Can you work these out from the model? Positions are in its coordinate system, mm. Face numbers are marked on the shaded views. A direction names the side the tool comes from. Give positions to 0.01 mm unless a question says otherwise; leave off trailing zeros. Loops run counter-clockwise (first coordinate to the right, second up) from the corner with the lowest first, then second, coordinate; pieces in that order, holes last.
from build123d import *

# Parameters (mm, degrees)
SALIENTE_EXTRUIR1_DEPTH    = 6
CORTAR_EXTRUIR1_DEPTH      = 22.970816212
CORTAR_EXTRUIR1_DEPTH_BACK = 22.970816212
CORTAR_EXTRUIR2_DEPTH      = 34.249140271
CORTAR_EXTRUIR2_DEPTH_BACK = 5.4
CROQUIS4_R                 = 2.5
CROQUIS5_R                 = 4.5
SALIENTE_EXTRUIR2_DEPTH    = 5.4


with BuildPart() as part:
    # Croquis2 → Saliente-Extruir1 (new, symmetric)
    with BuildSketch(Plane(origin=(0, 0, 0), x_dir=(0, 0, -1), z_dir=(1, 0, 0))):
        with BuildLine():
            Line((7.8, 9.244722598), (7.8, -1.675439815))
            ThreePointArc((7.8, -1.675439815), (7.349392081, -3.749814828), (6.078787323, -5.450297917))
            Line((6.078787323, -5.450297917), (-5.789489169, -15.758911763))
            Line((-5.789489169, -15.758911763), (-12.497767664, -8.035690663))
            Line((-12.497767664, -8.035690663), (-9.521212677, -5.450297917))
            ThreePointArc((-9.521212677, -5.450297917), (-8.250607919, -3.749814828), (-7.8, -1.675439815))
            Line((-7.8, -1.675439815), (-7.8, 9.244722598))
            ThreePointArc((-7.8, 9.244722598), (0, 17.044722598), (7.8, 9.244722598))
        make_face()
    extrude(amount=SALIENTE_EXTRUIR1_DEPTH, both=True)

    # Croquis3 → Cortar-Extruir1 (cut, two sides: drawn at the far end of the back side and taken through both)
    with BuildSketch(Plane.XY.offset(-CORTAR_EXTRUIR1_DEPTH_BACK)):
        with BuildLine():
            Line((-6, 17.044722598), (-0.5698886, 15.224393056))
            ThreePointArc((-0.5698886, 15.224393056), (2.264862856, 13.331444594), (3.751873119, 10.264219435))
            Line((3.751873119, 10.264219435), (6, -1.675439815))
            Line((6, -1.675439815), (6, 17.044722598))
            Line((6, 17.044722598), (-6, 17.044722598))
        make_face()
    extrude(amount=CORTAR_EXTRUIR1_DEPTH + CORTAR_EXTRUIR1_DEPTH_BACK, mode=Mode.SUBTRACT)

    # Croquis4 → Cortar-Extruir2 (cut, two sides: drawn at the far end of the back side and taken through both)
    with BuildSketch(Plane(origin=(0, -9.642863705, 11.101800332), x_dir=(1, 0, 0), z_dir=(0, -0.6557574645123035, 0.7549716204841048)).offset(-CORTAR_EXTRUIR2_DEPTH_BACK)):
        with Locations(Location((0, -2.991213966, 0), (0, 0, 90))):
            Circle(CROQUIS4_R)
    extrude(amount=CORTAR_EXTRUIR2_DEPTH + CORTAR_EXTRUIR2_DEPTH_BACK, mode=Mode.SUBTRACT)

    # Croquis5 → Saliente-Extruir2 (add)
    with BuildSketch(Plane.ZY.offset(6)):
        with Locations(Location((0, 9.244722598, 0), (0, 0, 180))):
            Circle(CROQUIS5_R)
    extrude(amount=SALIENTE_EXTRUIR2_DEPTH)


solid = part.part
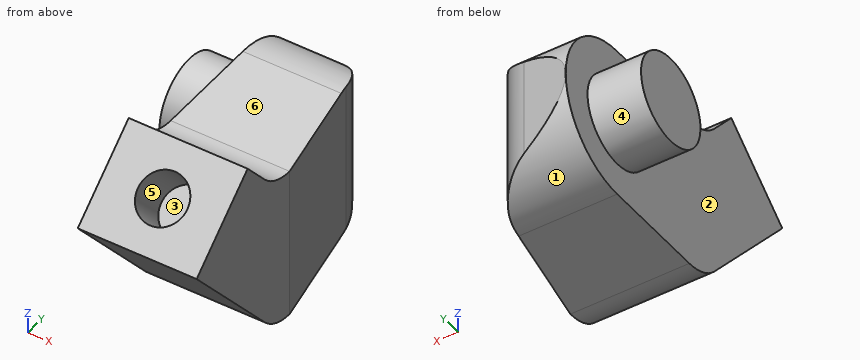
(1) Suppose I cut it at D-D on x = 5. List the corners of the cut face in (y, z) for me.
Returned:
outline: (-15.76, 5.79) - (-5.45, -6.08) arc R5 ccw to (-1.68, -7.8) - (3.64, -7.8) - (3.64, 7.8) - (-1.68, 7.8) arc R5 cw to (-5.45, 9.52) - (-8.04, 12.5) - close
(2) Which directions (+Z, -Z, +X, -X, +Y, -Y) give clear straight access to the entire face, cutting with the end or side of a thin tool? Please do the marked faces 4, 5 and 6.
Returned:
face 4: -X
face 5: none
face 6: +Z, +X, -X, +Y
(3) Suppose I cut it at B-B on x = -8.75. List the corners of the cut face in (y, z) for me, plus the area to 3 significant figures.
Returned:
outline: circle Ø9 at (9.24, 0)
area: 63.6 mm2
(4) Suppose I cut it at A-A on z = -2.5. List the corners of the cut face in (x, y) for me, plus the area to 3 significant figures.
Returned:
outline: (-11.4, 5.5) - (-6, 5.5) - (-6, -8.56) - (6, -8.56) - (6, -1.68) - (3.75, 10.26) arc R6.5 ccw to (-0.57, 15.22) - (-4.77, 16.63) - (-6, 16.63) - (-6, 12.99) - (-11.4, 12.99) - close
area: 299 mm2
(5) Thinking about a two-plate mould opening in Y: for the marked faces 1, 2 and 3, which applies, pulls with the +Y half, pulls with the -Y half, needs draft (parallel to the pull), parting line crosses it, or undercut?
Returned:
face 1: pulls with the +Y half
face 2: needs draft
face 3: undercut
(6) Please list where these lines run through material, in increasing order: probe 1 along X at (y, z) = (-3.5, 2.75); probe 2 along Z at (x, y) = (-1, 5); probe 3 along X at (y, z) = (-10, 4).
Returned:
probe 1: x = -6 to 6
probe 2: z = -7.8 to 7.8
probe 3: x = -6 to -1.58, 1.58 to 6
(7) Suppose I cut it at C-C on y = -6. List the corners of the cut face in (x, z) for me.
Returned:
outline: (-6, -5.45) - (6, -5.45) - (6, 10.15) - (-6, 10.15) - close
(8) Will these pins go through, and if not, where does the flat tip stop? P1, Ø1, axis at y = -2.5, z = 7.5, coming from the -X side; P2, Ø2, axis at x = 4, z = 5, coming from the +Y side; P3, Ø8.5, axis at x = 1, y = 6.5, coming from the +Z side.
Returned:
P1: stops at x = -6
P2: stops at y = 12.3
P3: stops at z = 7.8
